Source: CAD feature listing. Evaluate the final solid. Frame: model axes, mm. A direction names the side the tool comes from. Round coordinates to 2 decimals unless told otherwise and drop trailing zeros. Loops run counter-clockwise (first coordinate to the right, second up) from the corner with the lowest first, then second, coordinate; pieces in that order, holes last.
(1) Material intervals for probe 1 along X at (y, z) = (-2.5, 12); probe 2 along Z at (x, y) = (-35, 29); probe 3 along X at (y, z) = (29, 86), sorted ascending.
(2) Section D-D, the plane y = 7. Return the cut outline in (x, z).
(3) Section B-B, the plane y = -18.5. Return the cut outline in (x, z).
(4) Section C-C, the plane x = 241.5. Return the cut outline in (y, z), plus the area to 3 significant figures.
(5) Mould query, pull axis X, two halves, no side actions, for faces 1 (the flat face through (-217.729, 1, -13)), 2 (the flat face through (360.618, -1, -13)), 3 (the flat face through (66, 1, 0)), 4 (the flat face through (359, 1, 114.3)). Classes: pulls with the +X half, pulls with the -X half, needs draft (parallel to the pull), parting line crosses it, or undercut.
(6) Set-up query: faces 5 (the flat face through (379, 1, 0)), 6 (the flat face through (67, 1, -25.4)), 7 (the flat face through (-235, 1, 0)). Return all of +Z, -Z, +X, -X, +Y, -Y with unobstructed straight access to the full face (end or side cutting, diameter ignored); none if empty.
(7) First-contact query: pin 1 Ø13 at (x, y) = (379.5, 4) entering from -Z; pin 2 Ø1.5 at (x, y) = (-29.5, -21.5) entering from +Z; pin 3 Ø3 at (y, z) = (-1.5, 38.5) entering from +X; pin 4 Ø12.5 at (y, z) = (16, -6.5) entering from -X. Flat tips, straight axial feed; report the tip coordinate or a pass-through.
(8) Section A-A, the plane z = 23. Return the cut outline in (x, y) (3 decimals).
```python
from build123d import *

# Parameters (mm, degrees)
F1_DEPTH = 114.3
F2_DEPTH = 25.4


with BuildPart() as f1:
    # F0 (on Top) → F1 (new body)
    with BuildSketch(Plane.XY):
        with BuildLine():
            ThreePointArc((400.6691527557, 0), (387.8651300869, 29.8835920667), (357.3969989189, 41.2266540184))
            Line((357.3969989189, 41.2266540184), (360.6180139352, 41.2266540184))
            Line((360.6180139352, 41.2266540184), (360.6180139352, -41.2568514166))
            ThreePointArc((360.6180139352, -41.2568514166), (389.0095245682, -28.7498761286), (400.6691527557, 0))
        make_face()
        with BuildLine():
            Line((360.6180139352, 41.2266540184), (357.3969989189, 41.2266540184))
            ThreePointArc((357.3969989189, 41.2266540184), (318.1209665249, -0.3869410216), (358.1702915763, -41.2568514166))
            Line((358.1702915763, -41.2568514166), (360.6180139352, -41.2568514166))
            Line((360.6180139352, -41.2568514166), (360.6180139352, 41.2266540184))
        make_face()
    extrude(amount=F1_DEPTH)



with BuildPart() as f1b:
    # F0 (on Top) → F1, piece 2 (new body)
    with BuildSketch(Plane.XY):
        with BuildLine():
            Line((-217.7286934074, -41.2266540184), (-217.7286934074, 41.2266540184))
            ThreePointArc((-217.7286934074, 41.2266540184), (-261.0008472443, 0), (-217.7286934074, -41.2266540184))
        make_face()
        with BuildLine():
            ThreePointArc((-217.7286934074, -41.2266540184), (-189.8422551776, -28.4709773312), (-178.4508472443, 0))
            ThreePointArc((-178.4508472443, 0), (-189.8422551776, 28.4709773312), (-217.7286934074, 41.2266540184))
            Line((-217.7286934074, 41.2266540184), (-217.7286934074, -41.2266540184))
        make_face()
    extrude(amount=F1_DEPTH)


with BuildPart() as f1_1:
    add(f1.part)

    add(f1b.part)  # F2 merges F1b
    # F0 (on Top) → F2 (join)
    with BuildSketch(Plane.XY):
        with BuildLine():
            ThreePointArc((-217.7286934074, -41.2266540184), (-189.8422551776, -28.4709773312), (-178.4508472443, 0))
            ThreePointArc((-178.4508472443, 0), (-189.8422551776, 28.4709773312), (-217.7286934074, 41.2266540184))
            Line((-217.7286934074, 41.2266540184), (-217.7286934074, -41.2266540184))
        make_face()
        with BuildLine():
            ThreePointArc((-217.7286934074, 41.2266540184), (-189.8422551776, 28.4709773312), (-178.4508472443, 0))
            ThreePointArc((-178.4508472443, 0), (-189.8422551776, -28.4709773312), (-217.7286934074, -41.2266540184))
            Line((-217.7286934074, -41.2266540184), (-217.7286934074, -41.2568514166))
            Line((-217.7286934074, -41.2568514166), (358.1702915763, -41.2568514166))
            ThreePointArc((358.1702915763, -41.2568514166), (318.1209665249, -0.3869410216), (357.3969989189, 41.2266540184))
            Line((357.3969989189, 41.2266540184), (-217.7286934074, 41.2266540184))
        make_face()
        with BuildLine():
            Line((360.6180139352, 41.2266540184), (357.3969989189, 41.2266540184))
            ThreePointArc((357.3969989189, 41.2266540184), (318.1209665249, -0.3869410216), (358.1702915763, -41.2568514166))
            Line((358.1702915763, -41.2568514166), (360.6180139352, -41.2568514166))
            Line((360.6180139352, -41.2568514166), (360.6180139352, 41.2266540184))
        make_face()
    extrude(amount=-F2_DEPTH)


solid = f1_1.part
```
Output values:
1. probe 1: x = -260.93 to -178.53, 318.19 to 400.59
1. probe 2: z = -25.4 to 0
1. probe 3: x = -249.1 to -190.36, 330.02 to 388.76
2. outline: (-260.4, 0) - (-217.73, 0) - (-217.73, -25.4) - (360.62, -25.4) - (360.62, 0) - (400.07, 0) - (400.07, 114.3) - (318.72, 114.3) - (318.72, 0) - (-179.05, 0) - (-179.05, 114.3) - (-260.4, 114.3) - close
3. outline: (-256.62, 0) - (-217.73, 0) - (-217.73, -25.4) - (360.62, -25.4) - (360.62, 0) - (396.29, 0) - (396.29, 114.3) - (322.5, 114.3) - (322.5, 0) - (-182.83, 0) - (-182.83, 114.3) - (-256.62, 114.3) - close
4. outline: (-41.26, -25.4) - (41.23, -25.4) - (41.23, 0) - (-41.26, 0) - close
4. area: 2,100 mm2
5. face 1: pulls with the -X half
5. face 2: pulls with the +X half
5. face 3: undercut
5. face 4: needs draft
6. face 5: -Z, +X, +Y, -Y
6. face 6: -Z, +X, -X, +Y, -Y
6. face 7: -Z, -X, +Y, -Y
7. pin 1: stops at z = 0
7. pin 2: stops at z = 0
7. pin 3: stops at x = 400.67
7. pin 4: stops at x = -217.73
8. outline: circle Ø82.55 at (-219.726, 0); (358.17, -41.257) - (360.618, -41.257) arc R41.275 ccw (long way) to start
